Source: three-view drawing plus pictorial views. Frame: mm from the lowest corner of the part. Round coordinates to 2 decimals unless told otherwise and drop trailing zeros. Loops run counter-clockwise (first coordinate to the right, second up) from the corner with the lowest first, then second, coordinate; pieces in that order, holes last. Notation, with made-up numbers: (86.5, 39.5) -> (98.5, 39.5) arc R20 ccw to (98.5, 58.5) -> close; hole circle Ø3 at (19.25, 41). An arc over 180 degrees is marked (long way). Put each result on its own line as item: value. Start each with the question number.
1. Cut plane B-B (x = 63.5). Return the cut outline in (y, z).
2. Material intervals for L1, parallel to X at y = 19, z = 1.25 (1 decimal); L2, parallel to X at y = 7.62, z = 3.75 (1 decimal); L3, parallel to Y at x = 64.5, z = 4 (1 decimal), sorted ascending.
3. Contact query for flat-ended pins moving along their axis: pin 1 (3 mm diameter, centred on y = 33.5, z = 4.5, fed in from -X) (3 decimals); pin 2 (3 mm diameter, centred on y = 89, z = 4, fed in from -X); pin 3 (2 mm diameter, centred on y = 78.5, z = 2.5, fed in from +X). Output: stop coordinate, or through.
4. Cut plane A-A (y = 19.05). State how many separate pieces and enclosed holes the cut face has.
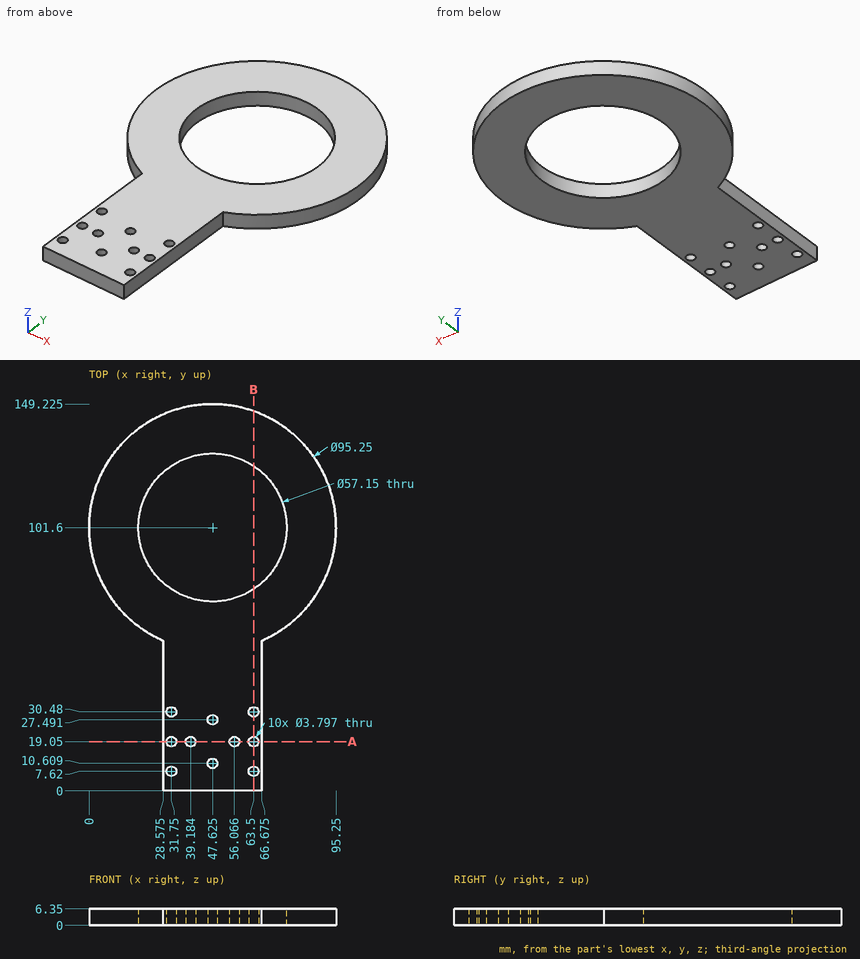
Solution:
1. outline: (0, 0) -> (5.72, 0) -> (5.72, 6.35) -> (0, 6.35) -> close; (9.52, 0) -> (17.15, 0) -> (17.15, 6.35) -> (9.52, 6.35) -> close; (20.95, 0) -> (28.58, 0) -> (28.58, 6.35) -> (20.95, 6.35) -> close; (32.38, 0) -> (77.84, 0) -> (77.84, 6.35) -> (32.38, 6.35) -> close; (125.36, 0) -> (146.5, 0) -> (146.5, 6.35) -> (125.36, 6.35) -> close
2. L1: x = 28.6 to 29.9, 33.6 to 37.3, 41.1 to 54.2, 58 to 61.6, 65.4 to 66.7
2. L2: x = 28.6 to 29.9, 33.6 to 61.6, 65.4 to 66.7
2. L3: y = 0 to 6, 9.2 to 17.4, 20.7 to 28.9, 32.1 to 78.5, 124.7 to 146.1
3. pin 1: stops at x = 28.575
3. pin 2: stops at x = 1.31
3. pin 3: stops at x = 89.81
4. separate pieces: 5
4. enclosed holes: 0
